Can you work these out from the model? Positions are in its coordinate system, mm. A direction names the side the tool comes from. Give positions to 0.01 mm unless a question says otherwise; leave off trailing zeros. Loops run counter-clockwise (first coordinate to the right, second up) from the corner with the lowest first, then second, coordinate; pieces in that order, holes last. Notation, with made-up numbers: M -22.75,0.5 L 5.25,0.5 A22 cw 5.25,24.5 Z; hole C -21,69 d2. An arc over 180 degrees is marked long. Answer as a JSON object with one key per item and string values.
Autodesk Inventor part; units mm, degrees
ref_plane "YZ Plane" through (0, 0, 0) normal (1, 0, 0) x (0, 1, 0)
ref_plane "XZ Plane" through (0, 0, 0) normal (0, 1, 0) x (-1, 0, 0)
ref_plane "XY Plane" through (0, 0, 0) normal (0, 0, 1) x (1, 0, 0)
sketch "Sketch1" plane through (0, 0, 0) normal (0, 0, 1) x (1, 0, 0)
  line L0 (7.9375, -7.9375) -> (-7.9375, -7.9375)
  line L1 (-7.9375, -7.9375) -> (-7.9375, 7.9375)
  line L2 (-7.9375, 7.9375) -> (7.9375, 7.9375)
  line L3 (7.9375, 7.9375) -> (7.9375, -7.9375)
  line L4 (-7.1437, -7.1438) -> (-7.1437, 7.1437)
  line L5 (-7.1437, 7.1437) -> (7.1437, 7.1438)
  line L6 (7.1437, 7.1438) -> (7.1438, -7.1437)
  line L7 (7.1438, -7.1437) -> (-7.1437, -7.1438)
  line L8 (0, 0) -> (5.5522, 0)
  point P0 (0, 0)
  point P1 (0, 0)
  point P2 (0, 0)
  dimension "d4" = 45
  dimension "d5" = 14.2875
  dimension "d6" = 15.875
extrude "Extrusion1" add sketch "Sketch1" along normal blind 203.2
sketch "Sketch2" plane through (-7.9375, 7.9375, 0) normal (0, 1, 0) x (1, 0, 0)
  line L0 (0, -203.2) -> (15.875, -203.2)
  line L1 (15.875, 0) -> (15.875, -203.2)
  line L2 (0, 0) -> (0, -203.2)
  line L3 (7.9375, -203.2) -> (7.9375, -257.0929)
  line L4 (7.9375, -193.675) -> (26.9875, -193.675) construction
  point P0 (7.9375, 0)
  point P1 (7.9375, -158.115)
  dimension "d27" = 9.525
  dimension "d30" = 35.56
hole "Hole1" at (0, 7.9375, 193.675) at (0, 7.9375, 158.115) direction (0, -1, 0) diameter 3.302 end through all
properties part number "Arm"
1) Suppose I cut it at A-A, the plane y = 0.5. Write out the boundary of the cut face in (x, z), and give its area (3 significant figures).
Answer list:
{"outline": "M -7.94,0 L -7.14,0 L -7.14,203.2 L -7.94,203.2 Z; M 7.14,0 L 7.94,0 L 7.94,203.2 L 7.14,203.2 Z", "area": "323 mm^2"}
2) Suppose I cut it at C-C, the plane z = 125.5. Write out the boundary of the cut face in (x, y), and give its area (3 significant figures).
Answer list:
{"outline": "M -7.94,-7.94 L 7.94,-7.94 L 7.94,7.94 L -7.94,7.94 Z; hole M -7.14,-7.14 L 7.14,-7.14 L 7.14,7.14 L -7.14,7.14 Z", "area": "47.9 mm^2"}
3) Please list where these lines run through material, in increasing order: line 1 along Z through (x, y) = (0, -7.7); line 2 along X through (y, z) = (1, 91). Write a range as from..to.
Answer list:
{"line 1": "0..156.46, 159.77..192.02, 195.33..203.2", "line 2": "-7.94..-7.14, 7.14..7.94"}
4) If we mould it in two halves opening along X, with no side actions, what happens to faces 1 (the flat face through (7.938, 0, 100)), 2 (the flat face through (-0.6, -7.6, 0)), 3 (the cylindrical face through (-0.073, 7.535, 192.026)), 4 (the flat face through (-7.938, 0, 100))? For each: +X half, -X half, draft (parallel to the pull), parting line (faces both ways), or undercut.
Answer list:
{"face 1": "+X half", "face 2": "draft", "face 3": "undercut", "face 4": "-X half"}
5) Will these pins go through, and if not, where does the flat tip stop? pin 1 Ø3 at (x, z) = (0, 193.675) entering from -Y; pin 2 Ø8 at (x, y) = (-6, 5.5) entering from +Z.
Answer list:
{"pin 1": "through", "pin 2": "z = 203.2"}
6) For faces 5 (the cylindrical face through (0.63, -7.55, 159.64)), 6 (the flat face through (-7.144, 0, 100)), which set-ups out of +Z, -Z, +X, -X, +Y, -Y let a thin tool reach every point of the face, with its end or its side?
Answer list:
{"face 5": "+Y, -Y", "face 6": "+Z, -Z"}
